from build123d import *

# Parameters (mm, degrees)
BOSS_EXTRU_1_DEPTH = 10


with BuildPart() as part:
    # Esquisse1 → Boss.-Extru.1 (new body)
    with BuildSketch(Plane(origin=(0, 0, 0), x_dir=(1, 0, 0), z_dir=(0, 1, 0))):
        with BuildLine():
            Line((0, -28), (-13, -28))
            Line((-13, -28), (-8, -33))
            Line((-8, -33), (-8, -30))
            Line((-8, -30), (-2, -30))
            Line((-2, -30), (-2, -34.467375879))
            Line((-2, -34.467375879), (0, -34.467375879))
            ThreePointArc((0, -34.467375879), (6, 0), (0, 34.467375879))
            Line((0, 34.467375879), (-2, 34.467375879))
            Line((-2, 34.467375879), (-2, 30))
            Line((-2, 30), (-8, 30))
            Line((-8, 30), (-8, 33))
            Line((-8, 33), (-13, 28))
            Line((-13, 28), (0, 28))
            ThreePointArc((0, 28), (4, 0), (0, -28))
        make_face()
    extrude(amount=BOSS_EXTRU_1_DEPTH)


solid = part.part
CAD build for the part. Positions are in the model's coordinates, mm. A direction names the side the tool comes from. Coordinates: 2 decimals unless noted, no trailing zeros. Loops run counter-clockwise (first coordinate to the right, second up) from the corner with the lowest first, then second, coordinate; pieces in that order, holes last. Notation, with made-up numbers: (33.25, -31) - (83.25, -31) arc R31 cw to (83.25, -2) - close; hole circle Ø6 at (28.25, -4). An arc over 180 degrees is marked (long way). Write item = value, one per line. Start each with the question number.
Q1. Cut at B-B, the plane y = 6. List the corners of the cut face in (x, z), then the cut area to 3 significant figures.
Q2. Flat gauge pins, fed straight in: pin 1 Ø0.9 at (y, z) = (5.5, -31) entering from +X; pin 2 Ø1.5 at (y, z) = (6, -4) entering from -X; pin 3 Ø5 at (y, z) = (7, 3.5) entering from -X; pin 4 Ø1.5 at (x, z) = (2.5, 2) entering from -Y. Where does each tip first touch, or does it go through?
Q3. Which spindle directions (+Z, -Z, +X, -X, +Y, -Y) get a long thin tool onto all of the face, cutting with end or side? Do faces 5 (the flat face through (-6, 5, 28)), 6 (the flat face through (4, 10, -8)), 7 (the flat face through (-5, 5, -30)), 8 (the flat face through (-8, 5, 32)). Say none if no direction does.
Q4. Cut at D-D, the plane z = -17.5. List the corners of the cut face in (x, y).
Q5. Pull direction X, two halves, no side cores. Call faces 1 (the cylindrical face through (6, 5, 0)), 2 (the flat face through (-2, 5, -32)), 3 (the flat face through (-11, 5, 30)), 4 (the flat face through (-1, 5, 34.467)): pulls with the +X half, pulls with the -X half, needs draft (parallel to the pull), parting line crosses it, or undercut.
Q6. Cut at C-C, the plane x = -9.75. List the corners of the cut face in (y, z).
Q7. Cut at A-A, the plane x = -5.5. List the corners of the cut face in (y, z), then the cut area to 3 significant figures.
Q8. Drill centre lines: L1, parallel to Z at x = -4.75, y = 8; L2, parallel to Z at x = -0.5, y = 5.25; L3, parallel to X at y = 9.75, z = -5.5. Where is each one in solid material? Low to high.
Computed:
q1.outline = (-13, -28) - (-8, -33) - (-8, -30) - (-2, -30) - (-2, -34.47) - (0, -34.47) arc R102 ccw to (0, 34.47) - (-2, 34.47) - (-2, 30) - (-8, 30) - (-8, 33) - (-13, 28) - (0, 28) arc R100 cw to (0, -28) - close
q1.area = 202 mm²
q2.pin_1 = 1.32
q2.pin_2 = 3.89
q2.pin_3 = 3.82
q2.pin_4 = through
q3.face_5 = -X, +Y, -Y
q3.face_6 = +Z, -Z, +X, -X, +Y
q3.face_7 = -Z, +Y, -Y
q3.face_8 = +Z, +Y, -Y
q4.outline = (2.46, 0) - (4.49, 0) - (4.49, 10) - (2.46, 10) - close
q5.face_1 = pulls with the +X half
q5.face_2 = undercut
q5.face_3 = pulls with the -X half
q5.face_4 = needs draft
q6.outline = (0, -31.25) - (10, -31.25) - (10, -28) - (0, -28) - close; (0, 28) - (10, 28) - (10, 31.25) - (0, 31.25) - close
q7.outline = (0, -30) - (10, -30) - (10, -28) - (0, -28) - close; (0, 28) - (10, 28) - (10, 30) - (0, 30) - close
q7.area = 40.0 mm²
q8.L1 = -30 to -28, 28 to 30
q8.L2 = -34.47 to -28, 28 to 34.47
q8.L3 = 3.85 to 5.85
